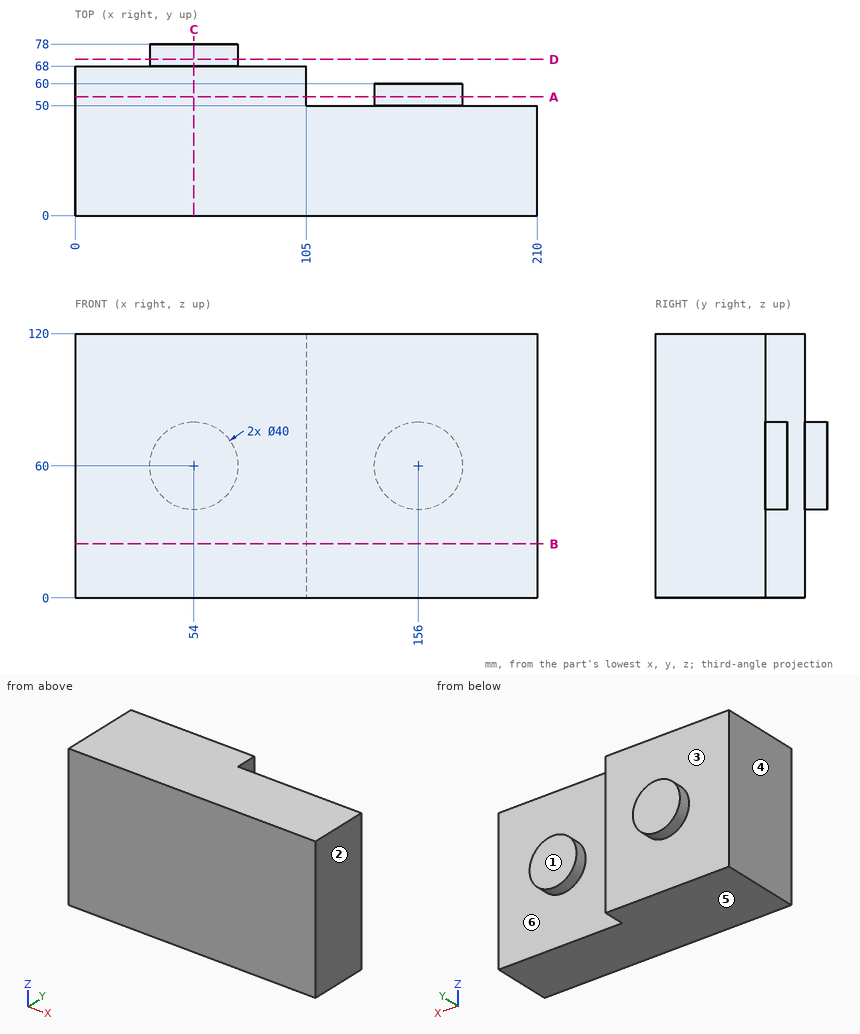
Drawing for the job (mm, zero at the part's lowest x, y, z). A direction names the side the tool comes from. Round coordinates to 2 decimals unless told otherwise and drop trailing zeros. Write each loop counter-clockwise with the first axis right and the second up, starting at its lowest first coordinate (ties: lowest second). Pieces come first, ordered by that corner, then holes. Notation, with made-up numbers: M 5.25,30 L 17.25,30 A29 cw 17.25,57 Z; hole C 14,-25 d4. An arc over 180 degrees is marked long. Answer as a JSON object with one key per item and string values. Group by question number.
(1) Drill centre lines: L1, parallel to X at y = 63, z = 45.5; L2, parallel to Y at x = 32, z = 112.5; L3, parallel to Y at x = 125.5, z = 69. Where is each one in solid material? Low to high.
(2) Cut at C-C (x = 54). Give the cut face in (y, z), and give its area (3 significant figures).
(3) Cut at A-A (y = 54). Give the cut face in (x, z), and give its area (3 significant figures).
(4) Mould opens along X. For the marked faces 4, 5 and 6 say: pulls with the +X half, pulls with the -X half, needs draft (parallel to the pull), parting line crosses it, or undercut.
(5) Cut at B-B (z = 24.5). Give the cut face in (x, y).
(6) Flat gauge pins, fed straight in: pin 1 (1 mm diameter, centred on x = 115.5, z = 82, fed in from -Y); pin 2 (4 mm diameter, centred on y = 66, z = 79, fed in from +X); pin 3 (12 mm diameter, centred on x = 113, z = 23.5, fed in from +Y); pin 4 (10 mm diameter, centred on x = 46.5, z = 33.5, fed in from +Y). Where does each tip first touch, or does it go through?
(7) Cut at D-D (y = 71). Give the cut face in (x, z).
(8) Which spindle directions (+Z, -Z, +X, -X, +Y, -Y) get a long thin tool onto all of the face, cutting with end or side? Do the marked faces 1, 2 and 3. Say none if no direction does.
Responses:
{
 "1": {"L1": "x = 0 to 105", "L2": "y = 0 to 68", "L3": "y = 0 to 50"},
 "2": {"outline": "M 0,0 L 68,0 L 68,40 L 78,40 L 78,80 L 68,80 L 68,120 L 0,120 Z", "area": "8,560 mm2"},
 "3": {"outline": "M 0,0 L 105,0 L 105,120 L 0,120 Z; C 156,60 d40", "area": "13,900 mm2"},
 "4": {"face 4": "pulls with the -X half", "face 5": "needs draft", "face 6": "undercut"},
 "5": {"outline": "M 0,0 L 210,0 L 210,50 L 105,50 L 105,68 L 0,68 Z"},
 "6": {"pin 1": "stops at y = 0", "pin 2": "stops at x = 105", "pin 3": "stops at y = 50", "pin 4": "stops at y = 68"},
 "7": {"outline": "C 54,60 d40"},
 "8": {"face 1": "+Z, -Z, +X, +Y", "face 2": "+Z, -Z, +X, +Y, -Y", "face 3": "+Y"}
}
